Build history of the part. All positions in model axes, mm. Face numbers are marked on the shaded views. A direction names the side the tool comes from. Round coordinates to 2 decimals unless told otherwise and drop trailing zeros. Write each loop counter-clockwise with the first axis right and the second up, starting at its lowest first coordinate (ties: lowest second). Pieces come first, ordered by that corner, then holes. Notation, with made-up numbers: (77.25, 30) -> (86.25, 30) arc R33 ccw to (86.25, 65) -> close; hole circle Ø3 at (-31, -4). An arc over 180 degrees is marked (long way). Return JSON: item names as keys, results as strings.
Autodesk Inventor part; units mm, degrees
ref_plane "YZ Plane" through (0, 0, 0) normal (1, 0, 0) x (0, 1, 0)
ref_plane "XZ Plane" through (0, 0, 0) normal (0, 1, 0) x (-1, 0, 0)
ref_plane "XY Plane" through (0, 0, 0) normal (0, 0, 1) x (1, 0, 0)
sketch "Skizze1" plane through (0, 0, 0) normal (0, 0, 1) x (1, 0, 0)
  line L0 (10, 15) -> (45.7133, 15) construction
  line L1 (10, 15) -> (10, -10) construction
  line L2 (37.1394, -10) -> (10, -10) construction
  line L3 (37.1394, -10) -> (37.1394, 14.1) construction
  line L4 (37.1394, 14.1) -> (45.7133, 14.1) construction
  line L5 (45.7133, 14.1) -> (45.7133, 15) construction
  line L6 (10, -10) -> (37.1394, -10)
  line L7 (37.1394, -10) -> (37.1394, 59.9176)
  line L8 (37.1394, 59.9176) -> (10, 59.9176)
  line L9 (10, 59.9176) -> (10, -10)
  point P0 (0, 0)
extrude "Extrusion1" add sketch "Skizze1" along normal blind 4
sketch "Skizze2" plane through (0, 0, 0) normal (0, 0, -1) x (-1, 0, 0)
  line L0 (-37.1394, 59.9176) -> (-10, 59.9176)
  line L1 (-10, 59.9176) -> (-37.1394, 59.9176)
  line L2 (-37.1394, 59.9176) -> (-37.1394, 62.9176)
  line L3 (-37.1394, 62.9176) -> (-10, 62.9176)
  line L4 (-10, 62.9176) -> (-10, 59.9176)
  point P0 (0, 0)
  dimension "d2" = 3
extrude "Extrusion2" add sketch "Skizze2" against normal blind 20
sketch "Skizze4" plane through (10, 62.9176, 0) normal (0, 1, 0) x (1, 0, 0)
  line L0 (27.1394, -4) -> (27.1394, -73.6709) construction
  line L1 (-71.0464, -73.5081) -> (53.1741, -73.5081) construction
  line L2 (53.1741, -72.4315) -> (53.1741, -73.5081) construction
  arc A0 (58.1741, -67.4315) -> (53.1741, -72.4315) centre (58.1741, -72.4315) ccw construction
  line L3 (62.2394, -67.4315) -> (58.1741, -67.4315) construction
  line L4 (62.2394, -59.1955) -> (62.2394, -67.4315) construction
  arc A1 (65.5394, -59.1955) -> (62.2394, -59.1955) centre (63.8894, -59.1955) ccw construction
  line L5 (65.5394, -67.4315) -> (65.5394, -59.1955) construction
  line L6 (81.2394, -67.4315) -> (65.5394, -67.4315) construction
  arc A2 (76.4341, -48.82) -> (81.2394, -67.4315) centre (125.2788, -46.1349) ccw construction
  arc A3 (76.4267, -48.4999) -> (76.4341, -48.82) centre (81.4265, -48.5455) ccw construction
  arc A4 (76.4267, -48.4999) -> (35.4184, -9) centre (29.7163, -55.9569) ccw construction
  line L7 (35.4184, -9) -> (-5, -9) construction
  line L8 (-5, -9) -> (-5, 9.9226) construction
  line L9 (-5, 9.9226) -> (-10, 9.9226) construction
  line L10 (-10, 9.9226) -> (-10, 9.9096) construction
  line L11 (-10, 9.9096) -> (-37.7867, 9.9096) construction
  arc A5 (-37.7867, 9.9096) -> (-54.9732, -24.6463) centre (-14.5965, -23.176) ccw construction
  arc A6 (-54.9732, -24.6463) -> (-71.0464, -73.5081) centre (23.4557, -77.5201) ccw construction
  arc A7 (-40.4634, -62.3724) -> (-28.4634, -62.3724) centre (-34.4634, -62.3724) ccw construction
  line L12 (-40.4634, -62.3724) -> (-40.4634, -47.5724) construction
  arc A8 (-28.4634, -47.5724) -> (-40.4634, -47.5724) centre (-34.4634, -47.5724) ccw construction
  line L13 (-28.4634, -47.5724) -> (-28.4634, -62.3724) construction
  arc A9 (-40.4634, -16.9802) -> (-28.4634, -16.9802) centre (-34.4634, -16.9802) ccw construction
  line L14 (-40.4634, -16.9802) -> (-40.4634, -2.1802) construction
  arc A10 (-28.4634, -2.1802) -> (-40.4634, -2.1802) centre (-34.4634, -2.1802) ccw construction
  line L15 (-28.4634, -2.1802) -> (-28.4634, -16.9802) construction
  line L16 (37.2394, -63.0832) -> (59.5394, -63.0832) construction
  line L17 (37.2394, -34.3078) -> (37.2394, -63.0832) construction
  arc A11 (59.5394, -34.3078) -> (37.2394, -34.3078) centre (48.3894, -34.3078) ccw construction
  line L18 (59.5394, -63.0832) -> (59.5394, -34.3078) construction
  arc A12 (62.2394, -38.1955) -> (65.5394, -38.1955) centre (63.8894, -38.1955) ccw construction
  line L19 (62.2394, -28.1955) -> (62.2394, -38.1955) construction
  arc A13 (65.5394, -28.1955) -> (62.2394, -28.1955) centre (63.8894, -28.1955) ccw construction
  line L20 (65.5394, -38.1955) -> (65.5394, -28.1955) construction
  arc A14 (34.5394, -59.1955) -> (31.2394, -59.1955) centre (32.8894, -59.1955) ccw construction
  line L21 (34.5394, -67.4315) -> (34.5394, -59.1955) construction
  line L22 (31.2394, -67.4315) -> (34.5394, -67.4315) construction
  line L23 (31.2394, -59.1955) -> (31.2394, -67.4315) construction
  arc A15 (31.2394, -38.1955) -> (34.5394, -38.1955) centre (32.8894, -38.1955) ccw construction
  line L24 (31.2394, -28.1955) -> (31.2394, -38.1955) construction
  arc A16 (34.5394, -28.1955) -> (31.2394, -28.1955) centre (32.8894, -28.1955) ccw construction
  line L25 (34.5394, -38.1955) -> (34.5394, -28.1955) construction
  line L26 (0, -4) -> (0, -78.5081) construction
  line L27 (27.1394, -20) -> (0, -20) construction
  circle A17 centre (13.5697, -15.0495) radius 2.1
  point P0 (-10, 0)
  dimension "d11" = 4.2
extrude "Extrusion4" cut sketch "Skizze4" against normal through all
sketch "Skizze5" plane through (10, -10, 0) normal (0, -1, 0) x (1, 0, 0)
  line L0 (0, 0) -> (27.1394, 0)
  line L1 (27.1394, 0) -> (27.1394, 4)
  line L2 (0, 4) -> (27.1394, 4)
  line L3 (0, 0) -> (0, 4)
  point P0 (-10, 0)
extrude "Extrusion5" add sketch "Skizze5" along normal blind 18
sketch "Skizze6" plane through (0, 0, 0) normal (0, 0, -1) x (-1, 0, 0)
  arc A0 (-23.2894, -22.5324) -> (-23.2894, -19.2324) centre (-23.2894, -20.8824) ccw construction
  arc A1 (-31.9894, -19.2324) -> (-31.9894, -22.5324) centre (-31.9894, -20.8824) ccw construction
  circle A2 centre (-31.9894, -20.8824) radius 1.65
  circle A3 centre (-23.2894, -20.8824) radius 1.65
  point P0 (0, 0)
extrude "Extrusion6" cut sketch "Skizze6" against normal through all
fillet "Rundung3" radius 2 7 edges at (37.1394, 17.4588, 0) (23.5697, -28, 0) (10, 17.4588, 0) (37.1394, 15.9588, 4) (23.5697, -28, 4) (23.5697, 62.9176, 0) (10, 15.9588, 4)
properties part number "Chain_fixture"
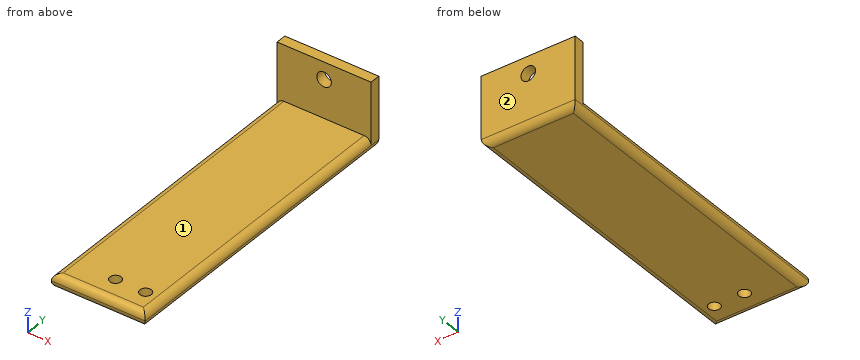
Q1. 3-axis set-ups, long thin cutter, end or side, ignore diameter. For the marked faces 1 and 2: which of +Z, -Z, +X, -X, +Y, -Y reach the whole face in a straight line?
Verdict:
{"face 1": "+Z, +X, -X, -Y", "face 2": "+Z, -Z, +X, -X, +Y"}
Q2. Pin check, flat tips, straight feed: pin 1 Ø10 at (x, y) = (33.5, 29.5) entering from +Z; pin 2 Ø4 at (x, z) = (33.5, 10.5) entering from -Y. Stop position of each tip, or through.
Verdict:
{"pin 1": "stops at z = 4", "pin 2": "stops at y = 59.92"}
Q3. Saw through at D-D on z = 7. List the corners of the cut face in (x, y).
Verdict:
{"outline": "(10, 59.92) -> (37.14, 59.92) -> (37.14, 62.92) -> (10, 62.92) -> close"}
Q4. Wall check: L1, parallel to Z at x = 19.5, y = 28; L2, parallel to Y at x = 14.5, z = 19.25; L3, parallel to X at y = -21, z = 1. Give the ranges that are in metal, low to high.
Verdict:
{"L1": "z = 0 to 4", "L2": "y = 59.92 to 62.92", "L3": "x = 10.27 to 21.64, 24.94 to 30.34, 33.64 to 36.87"}
